```python
from build123d import *

# Parameters (mm, degrees)
SKETCH1_R           = 38.1
BOSS_EXTRUDE1_DEPTH = 5.08
CUT_EXTRUDE1_DEPTH  = 98.514006601


with BuildPart() as part:
    # Sketch1 → Boss-Extrude1 (new body)
    with BuildSketch(Plane(origin=(0, 0, 0), x_dir=(1, 0, 0), z_dir=(0, 1, 0))):
        with Locations(Location((0, 0, 0), (0, 0, 270))):
            Circle(SKETCH1_R)
    extrude(amount=-BOSS_EXTRUDE1_DEPTH)

    # Sketch4 → Revolve1 (revolve)
    with BuildSketch(Plane.XY, mode=Mode.PRIVATE) as revolve1_sk:
        with BuildLine():
            Line((0, 0), (0, 76.19583579))
            Line((0, 76.19583579), (29.449785718, 76.19583579))
            ThreePointArc((29.449785718, 76.19583579), (13.250608801, 38.235955518), (28.786938765, 0))
            Line((28.786938765, 0), (0, 0))
        make_face()
    revolve(revolve1_sk.sketch.rotate(Axis((0, 0, 0), (0, 1, 0)), 90), axis=Axis((0, 0, 0), (0, 1, 0)))

    # Sketch5 → Cut-Extrude1 (cut, through all)
    with BuildSketch(Plane(origin=(0, -5.08, 0), x_dir=(-1, 0, 0), z_dir=(0, -1, 0))):
        Polygon((8.358877197, 0), (4.179438599, 7.239), (-4.179438599, 7.239), (-8.358877197, 0), (-4.179438599, -7.239), (4.179438599, -7.239), align=None)
    extrude(amount=-CUT_EXTRUDE1_DEPTH, mode=Mode.SUBTRACT)


solid = part.part
```
Check sheet for the modelled part. Datum: model origin and axes. Units: mm. A direction names the side the tool comes from. Round coordinates to 2 decimals unless told otherwise and drop trailing zeros. Loops run counter-clockwise (first coordinate to the right, second up) from the corner with the lowest first, then second, coordinate; pieces in that order, holes last. Notation, with made-up numbers: M 28.5,-11.75 L 71.5,-11.75 A8 cw 71.5,-5.75 Z; hole C -19.75,48.5 d9. An arc over 180 degrees is marked long. Answer as a JSON object with one key per item and string values.
1. Section check C-C (y = 68). Record the boundary of the cut face in (x, z), plus the area to 3 significant figures.
Reply:
{"outline": "C 0,0 d45.14; hole M -8.36,0 L -4.18,-7.24 L 4.18,-7.24 L 8.36,0 L 4.18,7.24 L -4.18,7.24 Z", "area": "1,420 mm²"}
2. Access from +Z, -Z, +X, -X, +Y, -Y to the whole of each face (thin tool, end or side, straight path). Record for faces 1 (the flat face through (-6.3, 34.99, -3.57)), 2 (the flat face through (1, -5.08, 8)).
Reply:
{"face 1": "+Y, -Y", "face 2": "+Z, -Z, +X, -X, -Y"}
3. Scan lines: line 1 (Z direction, x = -3, y = 58.5); line 2 (Z direction, x = -5, y = 62.5); line 3 (Y direction, x = 11.5, z = -21.5). Record each from-to range of solid material in increasing order.
Reply:
{"line 1": "z = -17.15 to -7.24, 7.24 to 17.15", "line 2": "z = -18.63 to -5.82, 5.82 to 18.63", "line 3": "y = -5.08 to 5.04, 70.5 to 76.2"}
4. Section check B-B (y = 2). Record the boundary of the cut face in (x, z), plus the area to 3 significant figures.
Reply:
{"outline": "C 0,0 d53.81; hole M -8.36,0 L -4.18,-7.24 L 4.18,-7.24 L 8.36,0 L 4.18,7.24 L -4.18,7.24 Z", "area": "2,090 mm²"}
5. Gauge pin test, flat ends, axial feed: P1, Ø9, axis at x = -0.5, y = 35.5, coming from the -Z side; P2, Ø4, axis at y = 23.5, z = -9.5, coming from the +X side; P3, Ø3, axis at y = 39, z = -9, coming from the +X side. Record the tip position at first contact, or that the pin passes through.
Reply:
{"P1": "stops at z = -13.67", "P2": "stops at x = 13.37", "P3": "stops at x = 10.94"}
6. Section check A-A (x = 0). Record the boundary of the cut face in (y, z), plus the area to 3 significant figures.
Reply:
{"outline": "M -5.08,-38.1 L 0,-38.1 L 0,-28.79 A53.67 cw 76.2,-29.45 L 76.2,-7.24 L -5.08,-7.24 Z; M -5.08,7.24 L 76.2,7.24 L 76.2,29.45 A53.67 cw 0,28.79 L 0,38.1 L -5.08,38.1 Z", "area": "1,980 mm²"}
